from build123d import *

# Parameters (mm, degrees)
PAD_DEPTH    = 2
SKETCH001_R  = 5.1
PAD001_DEPTH = 4
SKETCH003_R  = 1.4
PAD003_DEPTH = 2
PAD004_DEPTH = 4
FILLET_R     = 3
FILLET001_R  = 3
FILLET002_R  = 3
FILLET003_R  = 3
FILLET004_R  = 3
FILLET005_R  = 3
FILLET006_R  = 3
FILLET007_R  = 3


with BuildPart() as part:
    # Sketch → Pad (new body)
    with BuildSketch(Plane.XY):
        with BuildLine():
            Line((-36, 62.5), (36, 62.5))
            ThreePointArc((41, 57.5), (39.535534, 61.035534), (36, 62.5))
            Line((41, 57.5), (41, -57.5))
            ThreePointArc((36, -62.5), (39.535534, -61.035534), (41, -57.5))
            Line((36, -62.5), (-36, -62.5))
            ThreePointArc((-41, -57.5), (-39.535534, -61.035534), (-36, -62.5))
            Line((-41, -57.5), (-41, 57.5))
            ThreePointArc((-36, 62.5), (-39.535534, 61.035534), (-41, 57.5))
        make_face()
        with BuildLine():
            ThreePointArc((-30, 54.5), (-32.12132, 53.62132), (-33, 51.5))
            Line((-33, 39), (-33, 51.5))
            ThreePointArc((-33, 39), (-32.12132, 36.87868), (-30, 36))
            Line((30, 36), (-30, 36))
            ThreePointArc((30, 36), (32.12132, 36.87868), (33, 39))
            Line((33, 51.5), (33, 39))
            ThreePointArc((33, 51.5), (32.12132, 53.62132), (30, 54.5))
            Line((-30, 54.5), (30, 54.5))
        make_face(mode=Mode.SUBTRACT)
        with BuildLine():
            ThreePointArc((-30, -28), (-32.12132, -28.87868), (-33, -31))
            Line((-33, -51.5), (-33, -31))
            ThreePointArc((-33, -51.5), (-32.12132, -53.62132), (-30, -54.5))
            Line((30, -54.5), (-30, -54.5))
            ThreePointArc((30, -54.5), (32.12132, -53.62132), (33, -51.5))
            Line((33, -31), (33, -51.5))
            ThreePointArc((33, -31), (32.12132, -28.87868), (30, -28))
            Line((-30, -28), (30, -28))
        make_face(mode=Mode.SUBTRACT)
        with BuildLine():
            ThreePointArc((-30, 22), (-32.12132, 21.12132), (-33, 19))
            Line((-33, -11), (-33, 19))
            ThreePointArc((-33, -11), (-32.12132, -13.12132), (-30, -14))
            Line((30, -14), (-30, -14))
            ThreePointArc((30, -14), (32.12132, -13.12132), (33, -11))
            Line((33, 19), (33, -11))
            ThreePointArc((33, 19), (32.12132, 21.12132), (30, 22))
            Line((-30, 22), (30, 22))
        make_face(mode=Mode.SUBTRACT)
    extrude(amount=PAD_DEPTH)

    # Sketch001 → Pad001 (join)
    with BuildSketch(Plane(origin=(7.5, -20, 0), x_dir=(1, 0, 0), z_dir=(0, -1, 0))):
        with BuildLine():
            Line((10.4, 27), (10.4, 6))
            Line((33.5, 6), (10.4, 6))
            Line((33.5, 2), (33.5, 6))
            Line((-48.5, 2), (33.5, 2))
            Line((-48.5, 6), (-48.5, 2))
            Line((-25.4, 6), (-48.5, 6))
            Line((-25.4, 6), (-8.817564, 32.514577))
            ThreePointArc((10.4, 27), (2.868565, 36.996566), (-8.817564, 32.514577))
        make_face()
        with Locations((0, 27)):
            Circle(SKETCH001_R, mode=Mode.SUBTRACT)
    extrude(amount=PAD001_DEPTH)

    # Sketch003 → Pad003 (join)
    with BuildSketch(Plane(origin=(7.5, 30, 0), x_dir=(1, 0, 0), z_dir=(0, -1, 0))):
        with BuildLine():
            Line((33.5, 2), (-48.5, 2))
            Line((-48.5, 6), (-48.5, 2))
            Line((-25.4, 6), (-48.5, 6))
            Line((-8.817564, 32.514577), (-25.4, 6))
            ThreePointArc((10.4, 27), (2.868565, 36.996566), (-8.817564, 32.514577))
            Line((10.4, 27), (10.4, 6))
            Line((10.4, 6), (33.5, 6))
            Line((33.5, 6), (33.5, 2))
        make_face()
        with Locations((0, 27)):
            Circle(SKETCH003_R, mode=Mode.SUBTRACT)
        with Locations((-7, 27)):
            Circle(SKETCH003_R, mode=Mode.SUBTRACT)
        with Locations((0, 20)):
            Circle(SKETCH003_R, mode=Mode.SUBTRACT)
        with Locations((7, 27)):
            Circle(SKETCH003_R, mode=Mode.SUBTRACT)
        with Locations((0, 34)):
            Circle(SKETCH003_R, mode=Mode.SUBTRACT)
    extrude(amount=PAD003_DEPTH)

    # Sketch004 (on Face5 of Pad003) → Pad004 (join)
    with BuildSketch(Plane.XY.offset(2)):
        with BuildLine():
            Line((-36, 62.5), (36, 62.5))
            ThreePointArc((41, 57.5), (39.535534, 61.035534), (36, 62.5))
            Line((41, -57.5), (41, 57.5))
            ThreePointArc((36, -62.5), (39.535534, -61.035534), (41, -57.5))
            Line((-36, -62.5), (36, -62.5))
            ThreePointArc((-41, -57.5), (-39.535534, -61.035534), (-36, -62.5))
            Line((-41, 57.5), (-41, -57.5))
            ThreePointArc((-36, 62.5), (-39.535534, 61.035534), (-41, 57.5))
        make_face()
        with BuildLine():
            Line((-36, 60.5), (36, 60.5))
            ThreePointArc((39, 57.5), (38.12132, 59.62132), (36, 60.5))
            Line((39, 57.5), (39, -57.5))
            ThreePointArc((36, -60.5), (38.12132, -59.62132), (39, -57.5))
            Line((36, -60.5), (-36, -60.5))
            ThreePointArc((-39, -57.5), (-38.12132, -59.62132), (-36, -60.5))
            Line((-39, -57.5), (-39, 57.5))
            ThreePointArc((-36, 60.5), (-38.12132, 59.62132), (-39, 57.5))
        make_face(mode=Mode.SUBTRACT)
    extrude(amount=PAD004_DEPTH)

    # Fillet
    fillet_edges = [part.edges().sort_by_distance(p)[0] for p in [
        (-39, 4, 2),
    ]]
    fillet(fillet_edges, radius=FILLET_R)

    # Fillet001
    fillet001_edges = [part.edges().sort_by_distance(p)[0] for p in [
        (-39, -40.75, 2),
    ]]
    fillet(fillet001_edges, radius=FILLET001_R)

    # Fillet002
    fillet002_edges = [part.edges().sort_by_distance(p)[0] for p in [
        (0, -24, 2),
    ]]
    fillet(fillet002_edges, radius=FILLET002_R)

    # Fillet003
    fillet003_edges = [part.edges().sort_by_distance(p)[0] for p in [
        (1.5, 28, 2),
    ]]
    fillet(fillet003_edges, radius=FILLET003_R)

    # Fillet004
    fillet004_edges = [part.edges().sort_by_distance(p)[0] for p in [
        (1.5, -20, 2),
    ]]
    fillet(fillet004_edges, radius=FILLET004_R)

    # Fillet005
    fillet005_edges = [part.edges().sort_by_distance(p)[0] for p in [
        (39, 4, 2),
    ]]
    fillet(fillet005_edges, radius=FILLET005_R)

    # Fillet006
    fillet006_edges = [part.edges().sort_by_distance(p)[0] for p in [
        (0, 60.5, 2),
    ]]
    fillet(fillet006_edges, radius=FILLET006_R)

    # Fillet007
    fillet007_edges = [part.edges().sort_by_distance(p)[0] for p in [
        (0, 30, 2),
    ]]
    fillet(fillet007_edges, radius=FILLET007_R)


solid = part.part
Could you check a few things on this model? Use its own coordinates, in mm. A direction names the side the tool comes from. Give positions to 0.01 mm unless a question says otherwise; leave off trailing zeros. Order: outer loops, then holes, each group sorted by start corner. A loop starts at its lowest first (then second) coordinate and runs counter-clockwise, first axis right, second up.
Item 1: For faces 4 (the face through (3, -20, 15)), 5 (the face through (7.197, 29.014, 18.633)), 6 (the face through (-32.1, 21.14, 0.99)), 7 (the face through (10.549, 29.014, 36.943)), which set-ups out of +Z, -Z, +X, -X, +Y, -Y let a thin tool reach every point of the face, with its end or its side?
Item 2: If we section it at A-A, the plane x = 23: Count the separate pieces of the cut face and the enclosed holes in it, plus the area to 3 significant figures.
Item 3: If we mould it in two halves opening along Z, with no side actions, what happens to faces 1 (the face through (32.14, 53.6, 0.99)), 2 (the face through (6.394, -21.972, 22.021)), 3 (the face through (-0.5, 30.86, 2.9))? For each: pulls with the +Z half, pulls with the -Z half, needs draft (parallel to the pull), parting line crosses it, or undercut.
Item 4: If we section it at D-D, the plane z = 12: Write out the boundary of the cut face in (x, y), plus the area to 3 significant figures.
Item 5: If we section it at B-B, the plane y = 46: Write out the boundary of the cut face in (x, z).
Item 6: If we section it at C-C, the plane z = 34: Write out the boundary of the cut face in (x, y), plus the area to 3 significant figures.
Item 7: I need wall thicknesses on line 1 (Z direction, x = 7.5, y = 29.1); line 2 (Y direction, x = -18.5, z = 5.5); line 3 (Y direction, x = 4, z = 4). Which ranges of each line are inside material? Lowest first, please.
Item 8: I'm going to push flat-ended pins straight in: pin 1 (1 mm diameter, centred on x = 6, z = 31.5, fed in from -Y); pin 2 (6 mm diameter, centred on x = 7.5, z = 27, fed in from -Y); pin 3 (4 mm diameter, centred on x = -31, y = 26.5, fed in from +Z). Where does each tip first touch, or does it pass through?
Values:
1. face 4: +Z
1. face 5: +Y
1. face 6: +Z, -Z
1. face 7: +Z, +Y, -Y
2. separate pieces: 4
2. enclosed holes: 0
2. area: 140 mm2
3. face 1: needs draft
3. face 2: undercut
3. face 3: pulls with the +Z half
4. outline: (-14.15, -24) - (17.9, -24) - (17.9, -20) - (-14.15, -20) - close; (-14.15, 28) - (17.9, 28) - (17.9, 30) - (-14.15, 30) - close
4. area: 192 mm2
5. outline: (-41, 0) - (-33, 0) - (-33, 2) - (-36, 2) arc R3 cw to (-39, 5) - (-39, 6) - (-41, 6) - close; (33, 0) - (41, 0) - (41, 6) - (39, 6) - (39, 5) arc R3 cw to (36, 2) - (33, 2) - close
6. outline: (-0.19, -24) - (15.19, -24) - (15.19, -20) - (-0.19, -20) - close; (-0.19, 28) - (6.1, 28) - (6.1, 30) - (-0.19, 30) - close; (8.9, 28) - (15.19, 28) - (15.19, 30) - (8.9, 30) - close
6. area: 86.7 mm2
7. line 1: z = 0 to 18.6, 21.4 to 25.6, 28.4 to 32.6, 35.4 to 37.4
7. line 2: y = -62.5 to -60.5, -24 to -20, 28 to 30, 60.5 to 62.5
7. line 3: y = -62.5 to -60.33, -24.17 to -19.83, 27.83 to 30.17, 60.33 to 62.5
8. pin 1: stops at y = -24
8. pin 2: stops at y = 28
8. pin 3: stops at z = 6
